Autodesk Inventor part; units mm, degrees
ref_plane "YZ Plane" through (0, 0, 0) normal (1, 0, 0) x (0, 1, 0)
ref_plane "XZ Plane" through (0, 0, 0) normal (0, 1, 0) x (-1, 0, 0)
ref_plane "XY Plane" through (0, 0, 0) normal (0, 0, 1) x (1, 0, 0)
sketch "Sketch1" plane through (0, 0, 0) normal (0, 1, 0) x (-1, 0, 0)
  line L0 (-110.2739, 0) -> (-55.137, 95.5)
  line L1 (-55.137, 95.5) -> (55.137, 95.5)
  line L2 (55.137, 95.5) -> (110.2739, 0)
  line L3 (110.2739, 0) -> (55.137, -95.5)
  line L4 (55.137, -95.5) -> (-55.137, -95.5)
  line L5 (-55.137, -95.5) -> (-110.2739, 0)
  line L6 (60.9105, -85.5) -> (116, -85.5)
  line L7 (116, -85.5) -> (116, 85.5)
  line L8 (116, 85.5) -> (60.9105, 85.5)
  point P0 (0, 0)
  point P1 (0, 0)
  point P2 (116, 0)
  dimension "d5" = 191
  dimension "d6" = 171
  dimension "d7" = 116
extrude "Extrusion1" add sketch "Sketch1" along normal mid plane 2.55
properties part number "PlayerTacticalMats_All" material "Paper"
Check sheet for the modelled part. Datum: model origin and axes. Units: mm. Round coordinates to 2 decimals unless told otherwise and drop trailing zeros. Write each loop counter-clockwise with the first axis right and the second up, starting at its lowest first coordinate (ties: lowest second). Pieces come first, ordered by that corner, then holes. Notation, with made-up numbers: (-22, 70.25) -> (30, 70.25) arc R24 cw to (30, 84.25) -> close; hole circle Ø9 at (32, 1.25). An arc over 180 degrees is marked (long way). Put each result on its own line as item: value.
(1) Go/stop test with a flat-tipped pin: pin 1 Ø1.5 at (y, z) = (0, -25.5) entering from +X. Record where the tip stops, or that it passes through.
Values found:
pin 1: stops at x = 95.98
(2) Sectioned sample at B-B (x = -90.5). Enter the section's corners in (y, z) (3 decimals), plus the area to 3 significant figures.
Values found:
outline: (-1.275, -85.5) -> (1.275, -85.5) -> (1.275, 85.5) -> (-1.275, 85.5) -> close
area: 436 mm^2
(3) Sectioned sample at A-A (y = -0.1). Enter the section's corners in (x, z), plus the area to 3 significant figures.
Values found:
outline: (-116, -85.5) -> (-60.91, -85.5) -> (-55.14, -95.5) -> (55.14, -95.5) -> (110.27, 0) -> (55.14, 95.5) -> (-55.14, 95.5) -> (-60.91, 85.5) -> (-116, 85.5) -> close
area: 36,800 mm^2
(4) Sectioned sample at C-C (z = 59.5). Enter the section's corners in (x, y) (3 decimals).
Values found:
outline: (-116, -1.275) -> (75.922, -1.275) -> (75.922, 1.275) -> (-116, 1.275) -> close
(5) Material ranges on line 1 (Z direction, x = -91.5, y = 0.2); line 2 (X direction, y = -0.75, z = 13.5); line 3 (X direction, y = 0.9, z = 59.5), recorded low to high.
Values found:
line 1: z = -85.5 to 85.5
line 2: x = -116 to 102.48
line 3: x = -116 to 75.92
